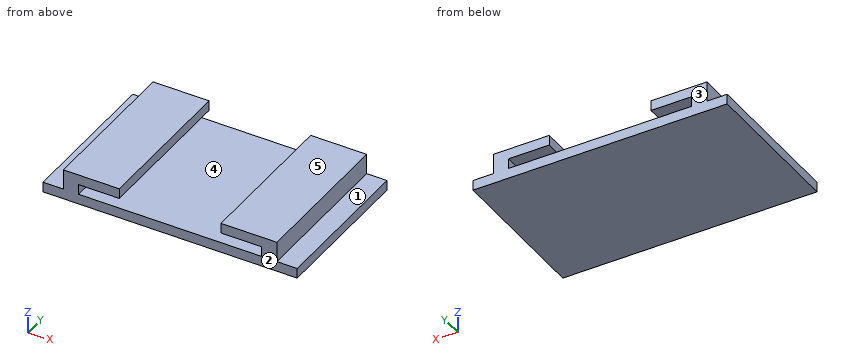
from build123d import *

# Parameters (mm, degrees)
SKETCH1_W               = 25
SKETCH1_H               = 15
BOSS_EXTRUDE1_DEPTH     = 1
SKETCH2_W               = 21
SKETCH2_H               = 15
BOSS_EXTRUDE2_DEPTH     = 3
CUT_EXTRUDE1_DEPTH      = 8.5
CUT_EXTRUDE1_DEPTH_BACK = 8.5


with BuildPart() as part:
    # Sketch1 → Boss-Extrude1 (new body)
    with BuildSketch(Plane.XY):
        Rectangle(SKETCH1_W, SKETCH1_H)
    extrude(amount=BOSS_EXTRUDE1_DEPTH)

    # Sketch2 → Boss-Extrude2 (add)
    with BuildSketch(Plane.XY):
        Rectangle(SKETCH2_W, SKETCH2_H)
    extrude(amount=BOSS_EXTRUDE2_DEPTH)

    # Sketch3 → Cut-Extrude1 (cut, two sides)
    with BuildSketch(Plane(origin=(0, 0, 0), x_dir=(1, 0, 0), z_dir=(0, 1, 0))) as cut_extrude1_sk:
        Polygon((-9, -2), (-5, -2), (-5, -3), (5, -3), (5, -2), (9, -2), (9, -1), (-9, -1), align=None)
    extrude(amount=CUT_EXTRUDE1_DEPTH, mode=Mode.SUBTRACT)
    extrude(cut_extrude1_sk.sketch, amount=-CUT_EXTRUDE1_DEPTH_BACK, mode=Mode.SUBTRACT)


solid = part.part
The model under review builds one solid part; all positions refer to its coordinate system, in mm. Face numbers are marked on the shaded views. A direction names the side the tool comes from. Round coordinates to 2 decimals unless told otherwise and drop trailing zeros. Order: outer loops, then holes, each group sorted by start corner. A loop starts at its lowest first (then second) coordinate and runs counter-clockwise, first axis right, second up. Notation, with made-up numbers: (-6, -39.75) -> (14, -39.75) arc R10 cw to (14, -24.75) -> close; hole circle Ø5 at (1.5, 17.25). An arc over 180 degrees is marked (long way). Return JSON: item names as keys, results as strings.
1. Insertion check: P1, Ø1.6, axis at y = 2.5, z = 2, coming from the +X side; P2, Ø1, axis at y = -4, z = 2.5, coming from the -X side; P3, Ø1.6, axis at x = -12, y = 1, coming from the +Z side. Each pin has a flat end and moves straight along its axis. Give the tip position at first contact, or say it passes through.
Answer block:
{"P1": "stops at x = 10.5", "P2": "stops at x = -10.5", "P3": "stops at z = 1"}
2. For the marked faces 1 and 2, list the 3-axis set-ups (+Z, -Z, +X, -X, +Y, -Y) from which the entire face can be reached by the end or side of a thin tool; tool diameter is ignored.
Answer block:
{"face 1": "+Z, +X, +Y, -Y", "face 2": "+Z, -Z, +X, -X, -Y"}
3. For L1, parallel to X at y = -1.75, z = 1.3; L2, parallel to X at y = -6.5, z = 2.3; L3, parallel to Z at x = -7.25, y = -3.75, list the stretches that pass through material, from the lowest coordinate up. Write a range as [from, to].
Answer block:
{"L1": "x = [-10.5, -9], [9, 10.5]", "L2": "x = [-10.5, -5], [5, 10.5]", "L3": "z = [0, 1], [2, 3]"}
4. The part is to be moulded in two halves that separate along Z. For the marked faces 3, 4 and 5, say which applies: +Z half, -Z half, draft (parallel to the pull), parting line (faces both ways), or undercut.
Answer block:
{"face 3": "draft", "face 4": "undercut", "face 5": "+Z half"}
5. Take a section at D-D (x = -3.75). Write out the cut boundary in (y, z), then the cut area to 3 significant figures.
Answer block:
{"outline": "(-7.5, 0) -> (7.5, 0) -> (7.5, 1) -> (-7.5, 1) -> close", "area": "15.0 mm²"}
6. Take a section at B-B (x = -8.75). Write out the cut boundary in (y, z), then the cut area to 3 significant figures.
Answer block:
{"outline": "(-7.5, 0) -> (7.5, 0) -> (7.5, 1) -> (-7.5, 1) -> close; (-7.5, 2) -> (7.5, 2) -> (7.5, 3) -> (-7.5, 3) -> close", "area": "30.0 mm²"}
7. Take a section at A-A (z = 2.4). Write out the cut boundary in (x, y).
Answer block:
{"outline": "(-10.5, -7.5) -> (-5, -7.5) -> (-5, 7.5) -> (-10.5, 7.5) -> close; (5, -7.5) -> (10.5, -7.5) -> (10.5, 7.5) -> (5, 7.5) -> close"}
8. Take a section at C-C (y = 2). Write out the cut boundary in (x, z).
Answer block:
{"outline": "(-12.5, 0) -> (12.5, 0) -> (12.5, 1) -> (10.5, 1) -> (10.5, 3) -> (5, 3) -> (5, 2) -> (9, 2) -> (9, 1) -> (-9, 1) -> (-9, 2) -> (-5, 2) -> (-5, 3) -> (-10.5, 3) -> (-10.5, 1) -> (-12.5, 1) -> close"}
